from build123d import *

# Parameters (mm, degrees)
SKETCH_1_W                  = 35.1
SKETCH_1_H                  = 36.1
SKETCH_1_W_2                = 19
SKETCH_1_H_2                = 9.5
EXTRUDE_1_DEPTH             = 4.5
CHAMFER_1_SIZE              = 2
SKETCH_4_W                  = 21
SKETCH_4_H                  = 11.5
SKETCH_4_W_2                = 19
SKETCH_4_H_2                = 9.5
EXTRUDE_2_DEPTH             = 100
SKETCH_5_W                  = 35.1
SKETCH_5_H                  = 36.1
SKETCH_5_W_2                = 19
SKETCH_5_H_2                = 9.5
EXTRUDE_3_DEPTH             = 4.5
CHAMFER_2_SIZE              = 2
PATTERN_LINEAR_1_COUNT      = 2
PATTERN_LINEAR_1_PITCH      = 29
PATTERN_LINEAR_1_COUNT_DIR2 = 2
PATTERN_LINEAR_1_PITCH_DIR2 = 30
HOLE_WIZARD_M42_D           = 4.5
HOLE_WIZARD_M42_CSINK_D     = 4.55
HOLE_WIZARD_M42_CSINK_ANGLE = 90


# Read off the part's stored shape, not the designer's step: Отверстие с зазором M41
with BuildPart() as part:
    # Эскиз1 → Бобышка-Вытянуть1 (new body)
    with BuildSketch(Plane(origin=(0, 0, 0), x_dir=(0, 0, -1), z_dir=(1, 0, 0))):
        Rectangle(SKETCH_1_W, SKETCH_1_H)
        Rectangle(SKETCH_1_W_2, SKETCH_1_H_2, mode=Mode.SUBTRACT)
    extrude(amount=EXTRUDE_1_DEPTH)

    # Фаска1
    chamfer_1_edges = [part.edges().sort_by_distance(p)[0] for p in [
        (2.25, -18.05, -17.55),
        (2.25, -18.05, 17.55),
        (2.25, 18.05, 17.55),
        (2.25, 18.05, -17.55),
    ]]
    chamfer(chamfer_1_edges, length=CHAMFER_1_SIZE)

    # Эскиз4 → Бобышка-Вытянуть2 (add)
    with BuildSketch(Plane(origin=(4.5, 0, 0), x_dir=(0, 0, -1), z_dir=(1, 0, 0))):
        Rectangle(SKETCH_4_W, SKETCH_4_H)
        Rectangle(SKETCH_4_W_2, SKETCH_4_H_2, mode=Mode.SUBTRACT)
    extrude(amount=EXTRUDE_2_DEPTH)

    # Эскиз5 → Бобышка-Вытянуть3 (add)
    with BuildSketch(Plane(origin=(104.5, 0, 0), x_dir=(0, 0, -1), z_dir=(1, 0, 0))):
        Rectangle(SKETCH_5_W, SKETCH_5_H)
        Rectangle(SKETCH_5_W_2, SKETCH_5_H_2, mode=Mode.SUBTRACT)
    extrude(amount=EXTRUDE_3_DEPTH)

    # Фаска2
    chamfer_2_edges = [part.edges().sort_by_distance(p)[0] for p in [
        (106.75, -18.05, -17.55),
        (106.75, 18.05, -17.55),
        (106.75, 18.05, 17.55),
        (106.75, -18.05, 17.55),
    ]]
    chamfer(chamfer_2_edges, length=CHAMFER_2_SIZE)

    # Отверстие с зазором M41 outline → Отверстие с зазором M41 (revolve, cut)
    with BuildSketch(Plane(origin=(0, 15, 14.5), x_dir=(0, 1, 0), z_dir=(0, 0, -1))):
        Polygon((2.25, 0.025), (2.25, 4.5), (0, 4.5), (0, 0), (2.275, 0), align=None)
    hole_wizard_m41 = revolve(axis=Axis((0, 15, 14.5), (1, 0, 0)), mode=Mode.SUBTRACT)

    # Линейный массив1: Hole Wizard M41 2 × 2
    with Locations(*[(0, -j * PATTERN_LINEAR_1_PITCH_DIR2, -i * PATTERN_LINEAR_1_PITCH) for i in range(PATTERN_LINEAR_1_COUNT) for j in range(PATTERN_LINEAR_1_COUNT_DIR2) if (i, j) != (0, 0)]):
        add(hole_wizard_m41, mode=Mode.SUBTRACT)

    # Отверстие с зазором M42 (through all)
    with Locations(Plane(origin=(109, 15, 14.5), x_dir=(0, 0, 1), z_dir=(1, 0, 0))):
        with Locations((0, 0), (-29, 0), (-29, 30), (0, 30)):
            CounterSinkHole(HOLE_WIZARD_M42_D / 2, HOLE_WIZARD_M42_CSINK_D / 2, counter_sink_angle=HOLE_WIZARD_M42_CSINK_ANGLE)


solid = part.part
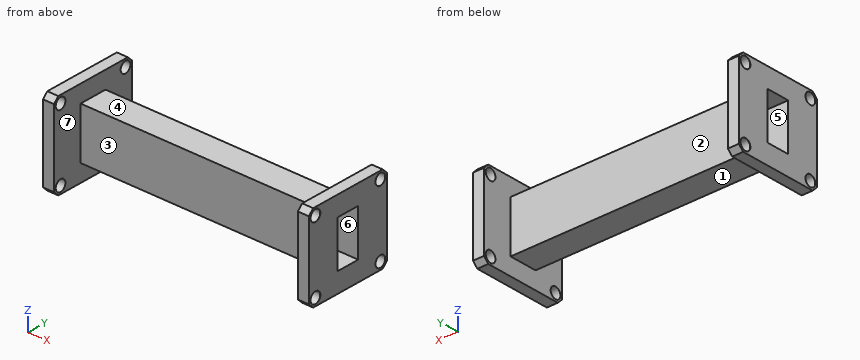
Input: part model. Units: mm. Frame: model coordinates. Face numbers are marked on the shaded views. A direction names the side the tool comes from. Give positions to 0.01 mm unless a question says otherwise; leave off trailing zeros. Loops run counter-clockwise (first coordinate to the right, second up) from the corner with the lowest first, then second, coordinate; pieces in that order, holes last. Notation, with made-up numbers: (48, 82) -> (56, 82) arc R8 ccw to (56, 95) -> close; hole circle Ø11 at (29.25, 45.5). An arc over 180 degrees is marked (long way). Answer as a JSON object with one key per item and string values. Group by question number.
Item 1: Pin query (flat end, axial travel): P1, Ø7.5, axis at x = 62, y = 0, coming from the -Z side; P2, Ø10.5, axis at x = 68, y = -2, coming from the +Z side; P3, Ø15, axis at x = 81, z = -4, coming from the +Y side. Return the tip coordinate at first contact, or that it passes through.
Item 2: Reachability of the marked faces 1, 2 and 3 from +Z, -Z, +X, -X, +Y, -Y: full face, straight path, thin tool, end or side. Return the list, or none.
Item 3: Cut plane A-A, the plane y = -15. State how many separate pieces and enclosed holes the cut face has, and give its area (3 significant figures).
Item 4: Cut plane B-B, the plane x = 62.5. Return the cut outline in (y, z).
Item 5: Line query: probe 1 along Y at (x, z) = (2.4, -14.5); probe 2 along Z at (x, y) = (1.65, 15); probe 3 along X at (y, z) = (-10, -12.5). Output: solid intervals per line, ascending.
Item 6: Pull-direction query (Z, two-part tool) for the marked faces 4, 5, 6 and 7; classes: released by +Z, released by -Z, zero draft, split by the parting line, or undercut.
Item 7: Cut plane C-C, the plane y = 2.5. Return the cut outline in (x, z).
Checks:
{
 "1": {"P1": "stops at z = -10.5", "P2": "stops at z = 10.5", "P3": "stops at y = 5.75"},
 "2": {"face 1": "-Z, +Y, -Y", "face 2": "+Z, -Z, +Y", "face 3": "+Z, -Z, -Y"},
 "3": {"separate pieces": "6", "enclosed holes": "0", "area": "235 mm²"},
 "4": {"outline": "(-5.75, -10.5) -> (5.75, -10.5) -> (5.75, 10.5) -> (-5.75, 10.5) -> close; hole (-4.75, -9.5) -> (4.75, -9.5) -> (4.75, 9.5) -> (-4.75, 9.5) -> close"},
 "5": {"probe 1": "y = -18.05 to -17.25, -12.75 to 12.75, 17.25 to 18.05", "probe 2": "z = -17.55 to -16.75, -12.25 to 12.25, 16.75 to 17.55", "probe 3": "x = 0 to 4.5, 104.5 to 109"},
 "6": {"face 4": "released by +Z", "face 5": "undercut", "face 6": "undercut", "face 7": "zero draft"},
 "7": {"outline": "(0, -17.55) -> (4.5, -17.55) -> (4.5, -10.5) -> (104.5, -10.5) -> (104.5, -17.55) -> (109, -17.55) -> (109, -9.5) -> (0, -9.5) -> close; (0, 9.5) -> (109, 9.5) -> (109, 17.55) -> (104.5, 17.55) -> (104.5, 10.5) -> (4.5, 10.5) -> (4.5, 17.55) -> (0, 17.55) -> close"}
}
